Build history of the part. All positions in model axes, mm. Face numbers are marked on the shaded views. A direction names the side the tool comes from. Give positions to 0.01 mm unless a question says otherwise; leave off trailing zeros. Loops run counter-clockwise (first coordinate to the right, second up) from the corner with the lowest first, then second, coordinate; pieces in that order, holes last. Notation, with made-up numbers: M 20.25,18 L 52.25,18 A16 ccw 52.25,24 Z; hole C 60.25,-18.5 d3. An arc over 180 degrees is marked long. Answer in a Markdown table with one row per item. Add a question column.
```python
from build123d import *

# Parameters (mm, degrees)
SKETCH1_W           = 25.4
SKETCH1_H           = 12.7
BOSS_EXTRUDE1_DEPTH = 2.54
CUT_EXTRUDE1_DEPTH  = 29.511429287
CHAMFER1_SIZE2      = 3.027054125
CHAMFER1_SIZE       = 2.54
SKETCH4_R           = 1.778
CUT_EXTRUDE2_DEPTH  = 1.27
CHAMFER3_SIZE       = 2.54
CHAMFER3_SIZE2      = 4.399409051
CHAMFER2_SIZE       = 5.08
CHAMFER2_SIZE2      = 4.385147389


with BuildPart() as part:
    # Sketch1 → Boss-Extrude1 (new body)
    with BuildSketch(Plane(origin=(0, 0, 0), x_dir=(1, 0, 0), z_dir=(0, 1, 0))):
        with Locations((12.7, -6.35)):
            Rectangle(SKETCH1_W, SKETCH1_H)
    extrude(amount=BOSS_EXTRUDE1_DEPTH)

    # Sketch2 → Cut-Extrude1 (cut, through all)
    with BuildSketch(Plane(origin=(0, 2.54, 0), x_dir=(1, 0, 0), z_dir=(0, 1, 0))):
        with BuildLine():
            ThreePointArc((22.098, -6.35), (20.32, -4.572), (18.542, -6.35))
            Line((18.542, -6.35), (22.098, -6.35))
        make_face()
        with BuildLine():
            Line((22.098, -6.35), (18.542, -6.35))
            ThreePointArc((18.542, -6.35), (20.32, -8.128), (22.098, -6.35))
        make_face()
        with BuildLine():
            ThreePointArc((15.748, -6.35), (13.97, -4.572), (12.192, -6.35))
            Line((12.192, -6.35), (15.748, -6.35))
        make_face()
        with BuildLine():
            Line((15.748, -6.35), (12.192, -6.35))
            ThreePointArc((12.192, -6.35), (13.97, -8.128), (15.748, -6.35))
        make_face()
    extrude(amount=-CUT_EXTRUDE1_DEPTH, mode=Mode.SUBTRACT)

    # Chamfer1
    chamfer1_edges = [part.edges().sort_by_distance(p)[0] for p in [
        (0, 2.54, 6.35),
    ]]
    chamfer1_side = [part.faces().sort_by_distance(p)[0] for p in [
        (0, 2.4892, 6.35),
    ]]
    chamfer(chamfer1_edges, length=CHAMFER1_SIZE - 0.0001, length2=CHAMFER1_SIZE2 - 0.0001, reference=chamfer1_side[0])  # a hair under: the kernel refuses the full size

    # Sketch4 → Cut-Extrude2 (cut)
    # profile 1 of 3: a face of its own
    with BuildSketch(Plane(origin=(0, 2.54, 0), x_dir=(1, 0, 0), z_dir=(0, 1, 0))):
        Polygon((17.145, -4.223618959), (13.97, -2.390531854), (10.541, -4.370265927), (10.541, -8.329734073), (13.97, -10.309468146), (17.145, -8.476381041), (16.891, -8.329734073), (16.891, -4.370265927), align=None)
        with Locations(Location((13.97, -6.35, 0), (0, 0, 270))):
            Circle(SKETCH4_R, mode=Mode.SUBTRACT)
    # profile 2 of 3: a face of its own
    with BuildSketch(Plane(origin=(0, 2.54, 0), x_dir=(1, 0, 0), z_dir=(0, 1, 0))):
        Polygon((20.32, -2.390531854), (17.145, -4.223618959), (17.399, -4.370265927), (17.399, -8.329734073), (17.145, -8.476381041), (20.32, -10.309468146), (23.749, -8.329734073), (23.749, -4.370265927), align=None)
        with Locations(Location((20.32, -6.35, 0), (0, 0, 270))):
            Circle(SKETCH4_R, mode=Mode.SUBTRACT)
    # profile 3 of 3: a face of its own
    with BuildSketch(Plane(origin=(0, 2.54, 0), x_dir=(1, 0, 0), z_dir=(0, 1, 0))):
        Polygon((17.399, -4.370265927), (17.145, -4.223618959), (16.891, -4.370265927), (16.891, -8.329734073), (17.145, -8.476381041), (17.399, -8.329734073), align=None)
    extrude(amount=-CUT_EXTRUDE2_DEPTH, mode=Mode.SUBTRACT)

    # Chamfer3
    chamfer3_edges = [part.edges().sort_by_distance(p)[0] for p in [
        (25.4, 1.27, 0),
        (25.4, 1.27, 12.7),
    ]]
    chamfer3_side = [part.faces().sort_by_distance(p)[0] for p in [
        (25.4, 1.27, 6.35),
    ]]
    chamfer(chamfer3_edges, length=CHAMFER3_SIZE, length2=CHAMFER3_SIZE2, reference=chamfer3_side[0])

    # Mirror1: part across plane


with BuildPart() as part_1:
    add(part.part)
    add(part.part.mirror(Plane(origin=(3.027054125, 2.54, 0), x_dir=(0, 0, 1), z_dir=(-0.6427876096865399, 0.7660444431189777, 0))))

    # Chamfer2
    chamfer2_edges = [part_1.edges().sort_by_distance(p)[0] for p in [
        (3.026954125, 2.54, 6.35),
    ]]
    chamfer2_side = [part_1.faces().sort_by_distance(p)[0] for p in [
        (4.587581401, 11.390189966, 0.257263255),
    ]]
    chamfer(chamfer2_edges, length=CHAMFER2_SIZE, length2=CHAMFER2_SIZE2, reference=chamfer2_side[0])


solid = part_1.part
```
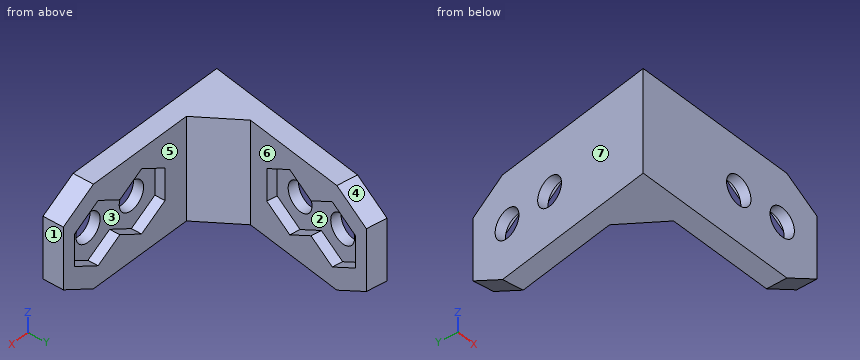
(1) Slice it at A-A, the plane z = 7.75. State how many separate pieces and enclosed holes the cut face has, then the cut area to 3 significant figures.
(2) Wall check: line 1 (Z direction, x = 20.32, y = 0.9); line 2 (X direction, y = 0.9, z = 6.35); line 3 (X direction, y = 0.6, z = 6.35). Give the ranges that are in metal, low to high.
(3) Slice it at C-C, the plane x = 8.5. Give the cut face in (y, z).
(4) Slice it at D-D, the plane z = 11.75. Give the cut face in (x, y).
(5) Pin check, flat tips, straight feed: pin 1 (5 mm diameter, centred on y = 21.5, z = 2, fed in from +X); pin 2 (5.5 mm diameter, centred on x = 13.97, z = 6.35, fed in from +Y); pin 3 (5 mm diameter, centred on y = 13, z = 7, fed in from -X). Stop position of each tip, or through.
(6) Pull direction Z, two halves, no side cores. Call the marked faces 1, 2, 3 and 4: +Z half, -Z half, draft (parallel to the pull), parting line (faces both ways), or undercut.
(7) Slice it at B-B, the plane x = 21.75. Give the cut face in (y, z), then the cut area to 3 significant figures.
(8) Tool access for the marked faces 5, 6 and 7: list every direction of +Z, -Z, +X, -X, +Y, -Y with a clear straight run to the whole face (end or side of a thin tool).
Solution:
| question | item | result |
|---|---|---|
| 1 | separate pieces | 5 |
| 1 | enclosed holes | 0 |
| 1 | area | 87.6 mm^2 |
| 2 | line 1 | 0 to 4.57, 8.13 to 12.7 |
| 2 | line 2 | 0.16 to 12.19, 15.75 to 18.54, 22.1 to 25.4 |
| 2 | line 3 | 0.11 to 12.19, 15.75 to 18.54, 22.1 to 25.4 |
| 3 | outline | M 0,0 L 2.54,0 L 2.54,12.7 L 0,12.7 Z |
| 4 | outline | M 0,0 L 22.65,0 L 22.65,2.54 L 7.41,2.54 L 3.91,7.54 L 6.43,21.86 L 3.93,22.3 Z |
| 5 | pin 1 | x = 6.81 |
| 5 | pin 2 | y = 1.27 |
| 5 | pin 3 | x = 1.85 |
| 6 | face 1 | draft |
| 6 | face 2 | undercut |
| 6 | face 3 | undercut |
| 6 | face 4 | +Z half |
| 7 | outline | M 0,0.43 L 2.54,0.43 L 2.54,3.22 L 1.27,3.22 L 1.27,5.29 L 0,5.29 Z; M 0,7.41 L 1.27,7.41 L 1.27,9.48 L 2.54,9.48 L 2.54,12.27 L 0,12.27 Z |
| 7 | area | 19.4 mm^2 |
| 8 | face 5 | +Z, -Z, +X, +Y |
| 8 | face 6 | +Z, -Z, +X |
| 8 | face 7 | +Z, -Z, -X, +Y |
